Verification items for this drawing (mm, ordinates from the low corner). Round coordinates to 2 decimals unless told otherwise and drop trailing zeros. Write each loop counter-clockwise with the first axis right and the second up, starting at its lowest first coordinate (ties: lowest second). Pieces come first, ordered by that corner, then holes.
Item 1: Cross-section at D-D (z = 12). Enter the section's corners in (x, y), then the cut area to 3 significant figures.
Item 2: Depth check by flat-ended pin: P1, Ø6, axis at y = 8.5, z = 6.5, coming from the +X side; P2, Ø4, axis at x = 48.5, z = 6.5, coming from the -Y side; P3, Ø3, axis at x = 40, z = 6, coming from the +Y side. Enter the tip coordinate at first touch or a pass-through.
Item 3: Cross-section at A-A (y = 16). Enter the section's corners in (x, z).
Item 4: Cross-section at C-C (x = 7). Enter the section's corners in (y, z), then the cut area to 3 significant figures.
Item 5: Draft check along Y on the marked faces 1 and 2. Enter one of: pulls with the +Y half, pulls with the -Y half, needs draft (parallel to the pull), parting line crosses it, or undercut.
Item 6: Cross-section at B-B (x = 40). Enter the section's corners in (y, z), then the cut area to 3 significant figures.
Item 7: Scan lines: probe 1 along Y at (x, z) = (40, 12.25); probe 2 along Z at (x, y) = (40, 0.9); probe 3 along X at (y, z) = (43, 14.25). Record each from-to range of solid material in increasing order.
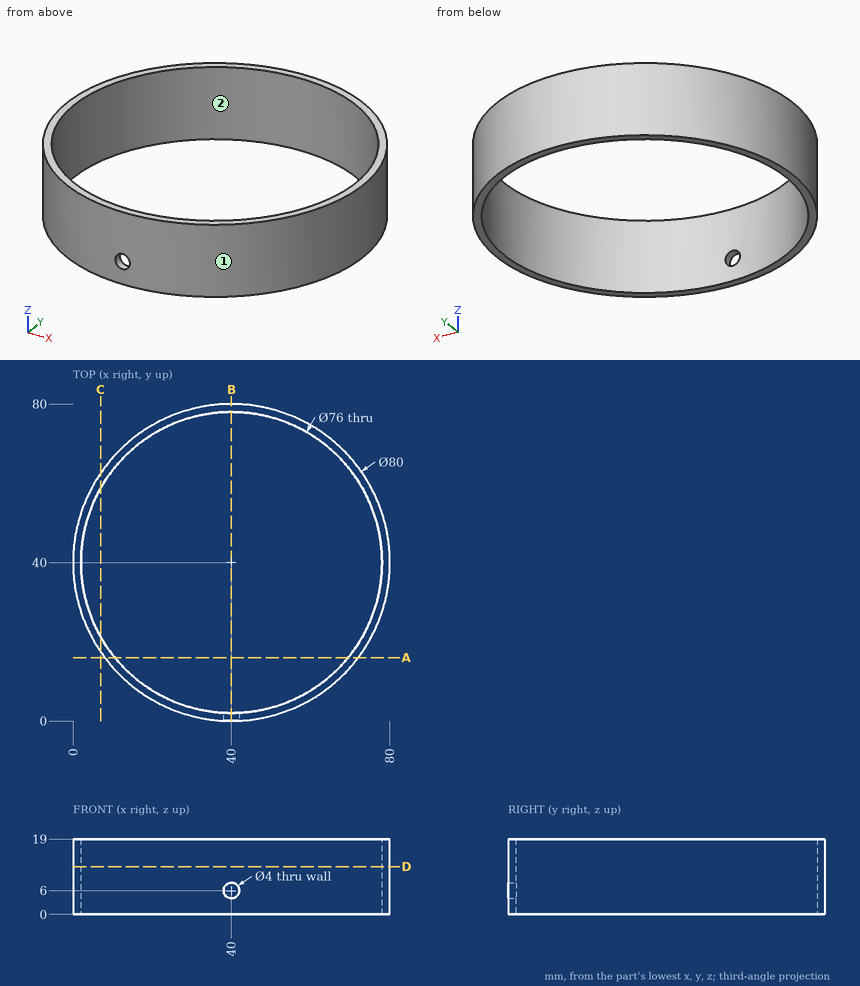
Resolved:
1. outline: circle Ø80 at (40, 40); hole circle Ø76 at (40, 40)
1. area: 490 mm2
2. P1: stops at x = 68.07
2. P2: stops at y = 0.53
2. P3: stops at y = 80
3. outline: (8, 0) - (10.54, 0) - (10.54, 19) - (8, 19) - close; (69.46, 0) - (72, 0) - (72, 19) - (69.46, 19) - close
4. outline: (17.39, 0) - (21.16, 0) - (21.16, 19) - (17.39, 19) - close; (58.84, 0) - (62.61, 0) - (62.61, 19) - (58.84, 19) - close
4. area: 143 mm2
5. face 1: parting line crosses it
5. face 2: undercut
6. outline: (0, 0) - (2, 0) - (2, 4) - (0, 4) - close; (0, 8) - (2, 8) - (2, 19) - (0, 19) - close; (78, 0) - (80, 0) - (80, 19) - (78, 19) - close
6. area: 68.0 mm2
7. probe 1: y = 0 to 2, 78 to 80
7. probe 2: z = 0 to 4, 8 to 19
7. probe 3: x = 0.11 to 2.12, 77.88 to 79.89
